```python
from build123d import *

# Parameters (mm, degrees)
BOSS_EXTRUDE1_DEPTH = 26.5
SKETCH4_W           = 6
SKETCH4_H           = 12
CUT_EXTRUDE2_DEPTH  = 19.5
FILLET2_R           = 0.3
FILLET3_R           = 0.3
BOSS_EXTRUDE3_DEPTH = 14.5
SKETCH8_R           = 2.15
CUT_EXTRUDE4_DEPTH  = 14.5
FILLET4_R           = 2
SKETCH9_W           = 53
SKETCH9_H           = 5
BOSS_EXTRUDE4_DEPTH = 13
SKETCH10_R          = 2
CUT_EXTRUDE5_DEPTH  = 10
FILLET9_R           = 5
SKETCH11_W          = 53
SKETCH11_H          = 5
BOSS_EXTRUDE5_DEPTH = 6.5
FILLET11_R          = 5
SKETCH12_W          = 57.342975089
SKETCH12_H          = 7.176836001
CUT_EXTRUDE6_DEPTH  = 5


with BuildPart() as part:
    # Sketch1 → Boss-Extrude1 (new body)
    with BuildSketch(Plane.XY):
        Polygon((-20.5, 2.5), (20.5, 2.5), (20.5, 22), (26.5, 22), (26.5, -2.5), (-26.5, -2.5), (-26.5, 22), (-20.5, 22), align=None)
    extrude(amount=BOSS_EXTRUDE1_DEPTH)

    # Sketch4 → Cut-Extrude2 (cut)
    with BuildSketch(Plane(origin=(0, 22, 0), x_dir=(1, 0, 0), z_dir=(0, 1, 0))):
        with Locations((-23.5, -6)):
            Rectangle(SKETCH4_W, SKETCH4_H)
        with Locations((23.5, -6)):
            Rectangle(SKETCH4_W, SKETCH4_H)
    extrude(amount=-CUT_EXTRUDE2_DEPTH, mode=Mode.SUBTRACT)

    # Fillet2
    fillet2_edges = [part.edges().sort_by_distance(p)[0] for p in [
        (20.5, 2.5, 19.25),
    ]]
    fillet(fillet2_edges, radius=FILLET2_R)

    # Fillet3
    fillet3_edges = [part.edges().sort_by_distance(p)[0] for p in [
        (-20.5, 2.5, 19.25),
    ]]
    fillet(fillet3_edges, radius=FILLET3_R)

    # Sketch7 → Boss-Extrude3 (add)
    with BuildSketch(Plane.XY.offset(26.5)):
        with BuildLine():
            Line((20.5, 19.707130751), (20.5, 15.492869249))
            ThreePointArc((20.5, 15.492869249), (27.9, 17.6), (20.5, 19.707130751))
        make_face()
        with BuildLine():
            Line((20.5, 9.507130751), (20.5, 5.292869249))
            ThreePointArc((20.5, 5.292869249), (27.9, 7.4), (20.5, 9.507130751))
        make_face()
    boss_extrude3 = extrude(amount=-BOSS_EXTRUDE3_DEPTH)

    # Sketch8 → Cut-Extrude4 (cut)
    with BuildSketch(Plane.XY.offset(26.5)):
        with Locations((23.9, 17.6)):
            Circle(SKETCH8_R)
        with Locations((23.9, 7.4)):
            Circle(SKETCH8_R)
    cut_extrude4 = extrude(amount=-CUT_EXTRUDE4_DEPTH, mode=Mode.SUBTRACT)

    # Mirror3: Boss-Extrude3, Cut-Extrude4 across plane
    add(boss_extrude3.mirror(Plane.ZY))
    add(cut_extrude4.mirror(Plane.ZY), mode=Mode.SUBTRACT)

    # Fillet4
    fillet4_edges = [part.edges().sort_by_distance(p)[0] for p in [
        (-23.35, 2.5, 12),
        (23.35, 2.5, 12),
    ]]
    fillet(fillet4_edges, radius=FILLET4_R)

    # Sketch9 → Boss-Extrude4 (add)
    with BuildSketch(Plane(origin=(0, 0, 0), x_dir=(-1, 0, 0), z_dir=(0, 0, -1))):
        Rectangle(SKETCH9_W, SKETCH9_H)
    extrude(amount=BOSS_EXTRUDE4_DEPTH)

    # Sketch10 → Cut-Extrude5 (cut)
    with BuildSketch(Plane(origin=(0, 2.5, 0), x_dir=(1, 0, 0), z_dir=(0, 1, 0))):
        with Locations((20, 5)):
            Circle(SKETCH10_R)
        with Locations((0, 5)):
            Circle(SKETCH10_R)
        with Locations((-20, 5)):
            Circle(SKETCH10_R)
    extrude(amount=-CUT_EXTRUDE5_DEPTH, mode=Mode.SUBTRACT)

    # Fillet9
    fillet9_edges = [part.edges().sort_by_distance(p)[0] for p in [
        (-26.5, 0, -13),
        (26.5, 0, -13),
    ]]
    fillet(fillet9_edges, radius=FILLET9_R)

    # Sketch11 → Boss-Extrude5 (add)
    with BuildSketch(Plane.XY.offset(26.5)):
        Rectangle(SKETCH11_W, SKETCH11_H)
    extrude(amount=BOSS_EXTRUDE5_DEPTH)

    # Fillet11
    fillet11_edges = [part.edges().sort_by_distance(p)[0] for p in [
        (-26.5, 0, 33),
        (26.5, 0, 33),
    ]]
    fillet(fillet11_edges, radius=FILLET11_R)

    # Sketch12 → Cut-Extrude6 (cut)
    with BuildSketch(Plane(origin=(0, 2.5, 0), x_dir=(1, 0, 0), z_dir=(0, 1, 0))):
        with Locations((-0.596167356, -30.088418001)):
            Rectangle(SKETCH12_W, SKETCH12_H)
    extrude(amount=-CUT_EXTRUDE6_DEPTH, mode=Mode.SUBTRACT)


solid = part.part
```
Verification items for the finished model (mm, model axes). A direction names the side the tool comes from. Give positions to 0.01 mm unless a question says otherwise; leave off trailing zeros. Order: outer loops, then holes, each group sorted by start corner. A loop starts at its lowest first (then second) coordinate and runs counter-clockwise, first axis right, second up. Notation, with made-up numbers: M 63,39.25 L 72,39.25 A19 cw 72,76.25 Z; hole C -10,12 d7. An arc over 180 degrees is marked long. Answer in a Markdown table with one row per item. Add a question column.
Item 1: Gauge pin test, flat ends, axial feed: pin 1 (5 mm diameter, centred on x = 0, z = -5, fed in from -Y); pin 2 (3.5 mm diameter, centred on y = 11.5, z = 18.5, fed in from +X); pin 3 (3.5 mm diameter, centred on x = 25, y = 10, fed in from -Z); pin 4 (5 mm diameter, centred on x = -19, z = 9.5, fed in from +Y). Record the tip position at first contact, or that the pin passes through.
Item 2: Mould release check, pull along X, two halves, no side actions. Record for faces 1 (the cylindrical face through (27.9, 7.4, 19.3)), 2 (the flat face through (-20.5, 13, 19)), 3 (the flat face through (0, 0, -13)): released by +X, released by -X, zero draft, split by the parting line, or undercut.
Item 3: Section check D-D, the plane z = 21. Enter the section's corners in (x, y).
Item 4: Section check C-C, the plane y = 7.4. Enter the section's corners in (x, z), and give its area (3 significant figures).
Item 5: Section check B-B, the plane y = 13.25. Enter the section's corners in (x, z).
Item 6: Tool access check on faces 4 (the flat face through (-24, 13, 12)), 5 (the flat face through (26.5, 21, 19)), 6 (the flat face through (-26.5, 1, 9)), 7 (the flat face through (0, 2.5, 6)). Record the directions out of +Z, -Z, +X, -X, +Y, -Y that give a thin tool (end or side, any length) a straight path to the whole face; none if there is none.
Item 7: Scan lines: probe 1 along Y at (x, z) = (-23.9, 16.25); probe 2 along X at (y, z) = (-1, -5); probe 3 along Z at (x, y) = (-20, 1.05). Record each from-to range of solid material in increasing order. Write a range as from..to.
Item 8: Section check A-A, the plane z = -5. Enter the section's corners in (x, y).
Filled sheet:
| question | item | result |
|---|---|---|
| 1 | pin 1 | stops at y = -2.5 |
| 1 | pin 2 | stops at x = 27.14 |
| 1 | pin 3 | stops at z = 12 |
| 1 | pin 4 | stops at y = 3.18 |
| 2 | face 1 | released by +X |
| 2 | face 2 | undercut |
| 2 | face 3 | zero draft |
| 3 | outline | M -26.5,-2.5 L 26.5,-2.5 L 26.5,4.36 A4 ccw 26.5,10.44 L 26.5,14.56 A4 ccw 26.5,20.64 L 26.5,22 L 20.5,22 L 20.5,2.8 A0.3 cw 20.2,2.5 L -20.2,2.5 A0.3 cw -20.5,2.8 L -20.5,22 L -26.5,22 L -26.5,20.64 A4 ccw -26.5,14.56 L -26.5,10.44 A4 ccw -26.5,4.36 Z; hole C -23.9,7.4 d4.3; hole C -23.9,17.6 d4.3; hole C 23.9,7.4 d4.3; hole C 23.9,17.6 d4.3 |
| 4 | outline | M -27.9,12 L -26.05,12 L -26.05,26.5 L -27.9,26.5 Z; M -21.75,12 L -20.5,12 L -20.5,26.5 L -21.75,26.5 Z; M 20.5,12 L 21.75,12 L 21.75,26.5 L 20.5,26.5 Z; M 26.05,12 L 27.9,12 L 27.9,26.5 L 26.05,26.5 Z |
| 4 | area | 89.9 mm^2 |
| 5 | outline | M -26.5,12 L -20.5,12 L -20.5,26.5 L -26.5,26.5 Z; M 20.5,12 L 26.5,12 L 26.5,26.5 L 20.5,26.5 Z |
| 6 | face 4 | -Z, +X, -X, +Y |
| 6 | face 5 | +Z, -Z, +X, +Y |
| 6 | face 6 | +Z, -Z, -X, -Y |
| 6 | face 7 | -Z, +Y |
| 7 | probe 1 | y = -2.5..5.25, 9.55..15.45, 19.75..22 |
| 7 | probe 2 | x = -26.5..-22, -18..-2, 2..18, 22..26.5 |
| 7 | probe 3 | z = -13..-7, -3..26.5 |
| 8 | outline | M -26.5,-2.5 L -22,-2.5 L -22,2.5 L -26.5,2.5 Z; M -18,-2.5 L -2,-2.5 L -2,2.5 L -18,2.5 Z; M 2,-2.5 L 18,-2.5 L 18,2.5 L 2,2.5 Z; M 22,-2.5 L 26.5,-2.5 L 26.5,2.5 L 22,2.5 Z |
